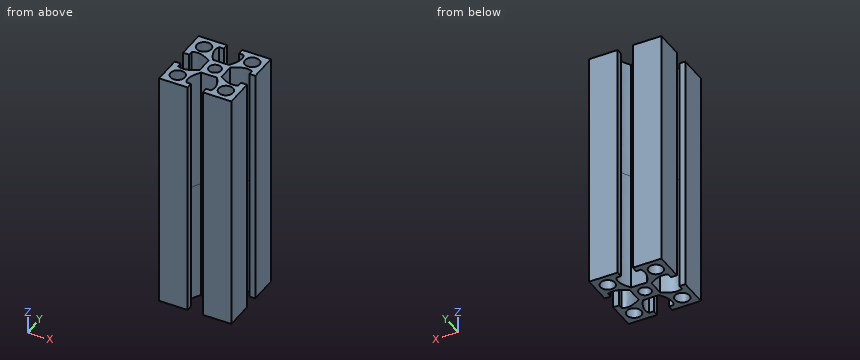
Autodesk Inventor part; units mm, degrees
ref_plane "YZ Plane" through (0, 0, 0) normal (1, 0, 0) x (0, 1, 0)
ref_plane "XZ Plane" through (0, 0, 0) normal (0, 1, 0) x (-1, 0, 0)
ref_plane "XY Plane" through (0, 0, 0) normal (0, 0, 1) x (1, 0, 0)
sketch "스케치1" plane through (0, 0, 0) normal (0, 0, 1) x (1, 0, 0)
  line L0 (3.335, 4.5) -> (0, 4.5)
  spline S0 degree 2 poles (3.335, 4.5) (6.7448, 9.4043) (5.1, 12.5) knots 0 0 0 1 1 1
  line L1 (4.5, 3.335) -> (4.5, 0)
  line L2 (-15, 15) -> (-15, -15)
  line L3 (-15, -15) -> (15, -15)
  line L4 (15, -15) -> (-15, 15) construction
  line L5 (-15, -15) -> (15, 15) construction
  line L6 (15, -3.15) -> (12.5, -3.15)
  line L7 (4.5, -3.335) -> (4.5, 0)
  line L8 (12.5, -3.15) -> (12.5, -5.1)
  spline S1 degree 2 poles (4.5, -3.335) (9.4043, -6.7448) (12.5, -5.1) knots 0 0 0 1 1 1
  line L9 (15, -15) -> (15, 15)
  circle A0 centre (10, -10) radius 3
  line L10 (15, 3.15) -> (12.5, 3.15)
  circle A1 centre (10, 10) radius 3
  spline S2 degree 2 poles (4.5, 3.335) (9.4043, 6.7448) (12.5, 5.1) knots 0 0 0 1 1 1
  line L11 (3.15, 12.5) -> (5.1, 12.5)
  line L12 (15, 15) -> (-15, 15)
  line L13 (0, 0) -> (0, 15) construction
  line L14 (3.15, 15) -> (3.15, 12.5)
  line L15 (-3.15, 15) -> (-3.15, 12.5)
  line L16 (-3.15, 12.5) -> (-5.1, 12.5)
  line L17 (-3.335, 4.5) -> (0, 4.5)
  spline S3 degree 2 poles (-3.335, 4.5) (-6.7448, 9.4043) (-5.1, 12.5) knots 0 0 0 1 1 1
  line L18 (-4.5, 3.335) -> (-4.5, 0)
  spline S4 degree 2 poles (-4.5, 3.335) (-9.4043, 6.7448) (-12.5, 5.1) knots 0 0 0 1 1 1
  line L19 (-12.5, 3.15) -> (-12.5, 5.1)
  line L20 (-15, 3.15) -> (-12.5, 3.15)
  circle A2 centre (-10, 10) radius 3
  circle A3 centre (0, 0) radius 2.5
  line L21 (-4.5, -3.335) -> (-4.5, 0)
  line L22 (-15, -3.15) -> (-12.5, -3.15)
  line L23 (-12.5, -3.15) -> (-12.5, -5.1)
  spline S5 degree 2 poles (-4.5, -3.335) (-9.4043, -6.7448) (-12.5, -5.1) knots 0 0 0 1 1 1
  line L24 (-3.335, -4.5) -> (0, -4.5)
  circle A4 centre (-10, -10) radius 3
  line L25 (3.335, -4.5) -> (0, -4.5)
  spline S6 degree 2 poles (-3.335, -4.5) (-6.7448, -9.4043) (-5.1, -12.5) knots 0 0 0 1 1 1
  line L26 (-3.15, -12.5) -> (-5.1, -12.5)
  line L27 (-3.15, -15) -> (-3.15, -12.5)
  spline S7 degree 2 poles (3.335, -4.5) (6.7448, -9.4043) (5.1, -12.5) knots 0 0 0 1 1 1
  line L28 (3.15, -12.5) -> (5.1, -12.5)
  line L29 (3.15, -15) -> (3.15, -12.5)
  line L30 (12.5, 3.15) -> (12.5, 5.1)
  point P0 (5.5866, 9.5531)
  point P1 (9.5531, -5.5866)
  point P2 (9.5531, 5.5866)
  point P3 (-5.5866, 9.5531)
  point P4 (-9.5531, 5.5866)
  point P5 (-9.5531, -5.5866)
  point P6 (-5.5866, -9.5531)
  point P7 (5.5866, -9.5531)
  dimension "d2" = 30
  dimension "d3" = 30
  dimension "d4" = 6
  dimension "d5" = 5
  dimension "d6" = 6.3
  dimension "d7" = 10.2
  dimension "d8" = 6.67
  dimension "d9" = 8
  dimension "d10" = 2.5
  dimension "d11" = 360
  dimension "d12" = 20
extrude "돌출1" add sketch "스케치1" along normal mid plane 100 contours S0 L11 L14 L12 L9 L10 L30 S2 L1 L7 S1 L8 L6 L3 L29 L28 S7 L25 L24 S6 L26 L27 L2 L22 L23 S5 L21 L18 S4 L19 L20 L15 L16 S3 L17 L0
equation "\"TransitionRadius\" = BendRadius"
properties part number "3030 Aluminium Profile 100mm"
The model under review builds one solid part; all positions refer to its coordinate system, in mm. Coordinates: 2 decimals unless noted, no trailing zeros. Write each loop counter-clockwise with the first axis right and the second up, starting at its lowest first coordinate (ties: lowest second). Pieces come first, ordered by that corner, then holes. Notation, with made-up numbers: (11, 4) -> (64, 4) arc R19 ccw to (64, 10) -> close; hole circle Ø6 at (-31.75, 44.5). An arc over 180 degrees is marked (long way). Answer in a Markdown table with one row per item.
1. We need section A-A, the plane x = 0. State the section outline as (y, z) points.
Answers below:
| item | result |
|---|---|
| outline | (-4.5, -50) -> (-2.5, -50) -> (-2.5, 50) -> (-4.5, 50) -> close; (2.5, -50) -> (4.5, -50) -> (4.5, 50) -> (2.5, 50) -> close |
2. We need section C-C, the plane z = -32. Give the number of separate pieces and of enclosed holes in the cut face, and give its area (3 significant figures).
Answers below:
| item | result |
|---|---|
| separate pieces | 1 |
| enclosed holes | 5 |
| area | 385 mm^2 |
3. Wall thickness on probe 1 along Y at (x, z) = (10, 18); probe 2 along Y at (x, z) = (7.5, -10); probe 3 along X at (y, z) = (-9.5, -28): over which ranges is each line inside the solid? List them lowest first. Write a range as [from, to].
Answers below:
| item | result |
|---|---|
| probe 1 | y = [-15, -13], [-7, -5.63], [5.63, 7], [13, 15] |
| probe 2 | y = [-15, -11.66], [-8.34, -5.02], [5.02, 8.34], [11.66, 15] |
| probe 3 | x = [-15, -12.96], [-7.04, -5.58], [5.58, 7.04], [12.96, 15] |
4. Clearance check with flat-ended pins moving along their axes: pin 1 Ø5.5 at (x, y) = (-10, -10) entering from -Z; pin 2 Ø1.5 at (x, z) = (-1.5, -25.5) entering from +Y. State where each tip first meets the part, or that it passes through.
Answers below:
| item | result |
|---|---|
| pin 1 | passes through |
| pin 2 | stops at y = 4.5 |
